```python
from build123d import *

# Parameters (mm, degrees)
EXTRUDE1_DEPTH     = 1403.35
SKETCH2_R          = 2.3876
SKETCH2_R_2        = 2.4257
CUT_EXTRUDE1_DEPTH = 1405.096860085
FILLET1_R          = 12.7


with BuildPart() as part:
    # Sketch1 → Extrude1 (new body)
    with BuildSketch(Plane.XY):
        Polygon((0, 0), (38.1, 0), (38.1, 3.175), (3.175, 3.175), (3.175, 25.4), (0, 25.4), align=None)
    extrude(amount=-EXTRUDE1_DEPTH)

    # Sketch2 → Cut-Extrude1 (cut, through all)
    with BuildSketch(Plane(origin=(0, 0, 0), x_dir=(1, 0, 0), z_dir=(0, 1, 0))):
        with Locations(Location((9.525, 254, 0), (0, 0, 180))):
            Circle(SKETCH2_R)
        with Locations(Location((28.575, 254, 0), (0, 0, 180))):
            Circle(SKETCH2_R)
        with Locations(Location((9.525, 1073.15, 0), (0, 0, 180))):
            Circle(SKETCH2_R)
        with Locations(Location((28.575, 1073.15, 0), (0, 0, 180))):
            Circle(SKETCH2_R)
        with Locations(Location((19.05, 19.05, 0), (0, 0, 180))):
            Circle(SKETCH2_R_2)
        with Locations(Location((19.05, 155.575, 0), (0, 0, 180))):
            Circle(SKETCH2_R_2)
        with Locations(Location((19.05, 428.625, 0), (0, 0, 180))):
            Circle(SKETCH2_R_2)
        with Locations(Location((19.05, 565.15, 0), (0, 0, 180))):
            Circle(SKETCH2_R_2)
        with Locations(Location((19.05, 701.675, 0), (0, 0, 180))):
            Circle(SKETCH2_R_2)
        with Locations(Location((19.05, 838.2, 0), (0, 0, 180))):
            Circle(SKETCH2_R_2)
        with Locations(Location((19.05, 974.725, 0), (0, 0, 180))):
            Circle(SKETCH2_R_2)
        with Locations(Location((19.05, 1247.775, 0), (0, 0, 180))):
            Circle(SKETCH2_R_2)
        with Locations(Location((19.05, 1384.3, 0), (0, 0, 180))):
            Circle(SKETCH2_R_2)
        with Locations(Location((28.575, 330.2, 0), (0, 0, 180))):
            Circle(SKETCH2_R)
        with Locations(Location((9.525, 330.2, 0), (0, 0, 180))):
            Circle(SKETCH2_R)
        with Locations(Location((28.575, 1149.35, 0), (0, 0, 180))):
            Circle(SKETCH2_R)
        with Locations(Location((9.525, 1149.35, 0), (0, 0, 180))):
            Circle(SKETCH2_R)
    extrude(amount=CUT_EXTRUDE1_DEPTH, mode=Mode.SUBTRACT)

    # Fillet1
    fillet1_edges = [part.edges().sort_by_distance(p)[0] for p in [
        (1.5875, 25.4, -1403.35),
        (1.5875, 25.4, 0),
    ]]
    fillet(fillet1_edges, radius=FILLET1_R)


solid = part.part
```
The listing builds one solid part. Answer for the finished solid, in the listing's coordinates (mm). A direction names the side the tool comes from. Coordinates: 2 decimals unless noted, no trailing zeros. Loops run counter-clockwise (first coordinate to the right, second up) from the corner with the lowest first, then second, coordinate; pieces in that order, holes last. Notation, with made-up numbers: (24, -18) - (58, -18) arc R32 cw to (58, 13) - close; hole circle Ø4 at (84.5, -33). An arc over 180 degrees is marked (long way). Use a Markdown table: item, result. Add a question column.
1) The part is cut by section A-A, the plane z = -1219. Give the vertices of the cut face in (x, y) (3 decimals).
2) Given pin 1 (4.5 mm diameter, centred on x = 9.525, z = -330.2, fed in from -Y); pin 2 (3 mm diameter, centred on y = 11.5, z = -1038, fed in from +X) (3 decimals); pin 3 (4 mm diameter, centred on x = 16.5, z = -168.5, fed in from +Y) (3 decimals), each flat-ended and moving along its own axis, determine where each tip first touches the part or whether it passes through.
3) The part is cut by section B-B, the plane y = 8.25. Give the vertices of the cut face in (x, z) (3 decimals), and give its area (3 significant figures).
4) Find the intervals of material crossed by line 1 (X direction, y = 1.55, z = -1149.35); line 2 (Z direction, x = 26.5, y = 2.5); line 3 (X direction, y = 1.2, z = -1384.3), in increasing order.
5) For faces 1 (the flat face through (0, 13, -692)), 2 (the flat face through (3.175, 14, -692)), determine the directions among +Z, -Z, +X, -X, +Y, -Y from which every point of the face is accessible in a straight line to the end or side of a thin tool.
Here are the results:
| question | item | result |
|---|---|---|
| 1 | outline | (0, 0) - (38.1, 0) - (38.1, 3.175) - (3.175, 3.175) - (3.175, 25.4) - (0, 25.4) - close |
| 2 | pin 1 | passes through |
| 2 | pin 2 | stops at x = 3.175 |
| 2 | pin 3 | stops at y = 3.175 |
| 3 | outline | (0, -1403.35) - (3.175, -1403.35) - (3.175, 0) - (0, 0) - close |
| 3 | area | 4,460 mm^2 |
| 4 | line 1 | x = 0 to 7.14, 11.91 to 26.19, 30.96 to 38.1 |
| 4 | line 2 | z = -1403.35 to -1150.53, -1148.17 to -1074.33, -1071.97 to -331.38, -329.02 to -255.18, -252.82 to 0 |
| 4 | line 3 | x = 0 to 16.62, 21.48 to 38.1 |
| 5 | face 1 | +Z, -Z, -X, +Y, -Y |
| 5 | face 2 | +Z, -Z, +X, +Y |
